Part model, mm, in its own coordinate system. Face numbers are marked on the shaded views. A direction names the side the tool comes from. Give positions to 0.01 mm unless a question says otherwise; leave off trailing zeros. Order: outer loops, then holes, each group sorted by start corner. A loop starts at its lowest first (then second) coordinate and runs counter-clockwise, first axis right, second up. Notation, with made-up numbers: (-32, 55.25) -> (24, 55.25) arc R29 ccw to (24, 91.25) -> close; hole circle Ø11 at (-3.75, 11). An arc over 180 degrees is marked (long way). Write item = value, one per line. Start each with the question number.
Item 1: Band-saw the part on B-B on x = -1.75. Write the cut outline in (y, z), plus the area to 3 significant figures.
Item 2: Band-saw the part on D-D on y = -1.5. Write the cut outline in (x, z).
Item 3: Drill centre lines: line 1 along Z through (x, y) = (4.75, 1.5); line 2 along Z through (x, y) = (8, 3.6); line 3 along X through (y, z) = (3.7, 0). Where is each one in solid material? Low to high.
Item 4: Tool access for the marked faces 4, 5 and 6: list every direction of +Z, -Z, +X, -X, +Y, -Y with a clear straight run to the whole face (end or side of a thin tool).
Item 5: Pull direction Z, two halves, no side cores. Call the marked faces 1, 2 and 3: +Z half, -Z half, draft (parallel to the pull), parting line (faces both ways), or undercut.
Item 6: Band-saw the part on C-C on z = 3. Write the cut outline in (x, y), plus the area to 3 significant figures.
Item 7: Band-saw the part on A-A on y = 0. Write the cut outline in (x, z), plus the area to 3 significant figures.
Item 8: Flat gauge pins, fed straight in: P1, Ø3, axis at y = -3, z = 2, coming from the -X side; P2, Ø2.5, axis at x = 6.5, z = -0.5, coming from the -Y side; P3, Ø3, axis at y = 2.5, z = 2.5, coming from the -X side; P4, Ø0.9, axis at y = 2, z = 1.5, coming from the -X side. Where does each tip first touch, or does it go through?
Autodesk Inventor part; units mm, degrees
ref_plane "Work Plane1" through (0, 0, -2.8) normal (0, 0, -1) x (-1, 0, 0)
ref_plane "Work Plane2" through (8, 0, 0) normal (1, 0, 0) x (0, 1, 0)
ref_plane "XZ Plane" through (0, 0, 0) normal (0, 1, 0) x (-1, 0, 0)
sketch "Sketch1" plane through (0, 0, 0) normal (0, 0, 1) x (1, 0, 0)
  circle A0 centre (0, 0) radius 4
  dimension "d0" = 8
extrude "Extrusion1" add sketch "Sketch1" along normal mid plane 8
sketch "Sketch2" plane through (0, 0, 4) normal (0, 0, 1) x (1, 0, 0)
  circle A0 centre (0, 0) radius 2.4
  line L0 (-2.2627, 0.8) -> (-0.8, 0.8)
  line L1 (-0.8, 0.8) -> (-0.8, 2.2627)
  line L2 (0.8, 2.2627) -> (0.8, 0.8)
  line L3 (0.8, 0.8) -> (2.2627, 0.8)
  line L4 (2.2627, -0.8) -> (0.8, -0.8)
  line L5 (0.8, -0.8) -> (0.8, -2.2627)
  line L6 (-0.8, -2.2627) -> (-0.8, -0.8)
  line L7 (-0.8, -0.8) -> (-2.2627, -0.8)
  dimension "d3" = 4.8
  dimension "d4" = 1.6
extrude "Extrusion2" cut sketch "Sketch2" against normal through all contours A0 L4 L5 L6 L7 L0 L1 L2 L3
ref_plane "Work Plane1" through (0, 0, -2.8) normal (0, 0, -1) x (-1, 0, 0)
sketch "Sketch3" plane through (0, 0, -2.8) normal (0, 0, -1) x (-1, 0, 0)
  circle A0 centre (0, 0) radius 4
  circle A1 centre (0, 0) radius 4
  circle A2 centre (0, 0) radius 3
  dimension "d8" = 6
extrude "Extrusion3" cut sketch "Sketch3" against normal blind 5.6
sketch "Sketch5" plane through (0, 0, 0) normal (0, 1, 0) x (-1, 0, 0)
  line L0 (-0.8, 4) -> (-0.8, -4)
  line L1 (0.8, 4) -> (0.8, -4)
  line L2 (4, 2.8) -> (-4, 2.8)
  line L3 (-0.8, -2.8) -> (0.8, -2.8)
  line L4 (0.8, -2.8) -> (0.8, 2.8)
  line L5 (0.8, 2.8) -> (-0.8, 2.8)
  line L6 (-0.8, 2.8) -> (-0.8, -2.8)
  point P0 (0, 0)
  point P1 (-1.518, -3.6)
  point P2 (4, -2.8)
  point P3 (4, -2.8)
extrude "Extrusion5" cut sketch "Sketch5" along normal through all both and the other way through all
fillet "Fillet1" radius 0.3 16 edges at (-0.8, 0.8, 0) (-0.8, -0.8, 0) (0.8, -0.8, 0) (0.8, 0.8, 0) (-2.2627, -0.8, 0) (-2.2627, 0.8, 0) (-0.8, 2.2627, 3.4) (0.8, 2.2627, 3.4) (2.2627, 0.8, 0) (2.2627, -0.8, 0) (0.8, -2.2627, 3.4) (-0.8, -2.2627, 3.4) (0.8, 2.2627, -3.4) (-0.8, 2.2627, -3.4) (0.8, -2.2627, -3.4) (-0.8, -2.2627, -3.4)
sketch "Sketch6" plane through (0, 0, 0) normal (0, 1, 0) x (-1, 0, 0)
  circle A0 centre (-8, 0) radius 2.5
  circle A1 centre (-8, 0) radius 4
  line L0 (-4, 2.8) -> (-4, 4)
  line L1 (-4, -4) -> (-4, -2.8)
  line L2 (-8, 4) -> (-8, -4) construction
  point P0 (0, 0)
  dimension "d22" = 5
  dimension "d23" = 8
  dimension "d24" = 8
extrude "Extrusion6" add sketch "Sketch6" along normal mid plane 8
sketch "Sketch7" plane through (8, 4, 0) normal (0, 1, 0) x (1, 0, 0)
  circle A0 centre (0, 0) radius 2.5
  circle A1 centre (0, 0) radius 4
  circle A2 centre (0, 0) radius 2.6667
  point P0 (-8, 0)
  dimension "d27" = 5.3333
extrude "Extrusion7" cut sketch "Sketch7" against normal blind 0.5333 contours A2
mirror "Mirror1" about plane through (0, 0, 0) normal (0, 1, 0) of "Extrusion7"
ref_plane "Work Plane2" through (8, 0, 0) normal (1, 0, 0) x (0, 1, 0)
sketch "Sketch8" plane through (8, 0, 0) normal (1, 0, 0) x (0, 1, 0)
  line L0 (-4, -2.6667) -> (-4, 2.6667)
  line L1 (-4, -4) -> (-4, 4)
  line L2 (4, 2.6667) -> (4, -2.6667)
  line L3 (4, 4) -> (4, -4)
  line L4 (4, 4) -> (-4, 4)
  line L5 (-4, 4) -> (-4, 2.8)
  line L6 (-4, 2.8) -> (4, 2.8)
  line L7 (4, 2.8) -> (4, 4)
  line L8 (-4, -4) -> (4, -4)
  line L9 (4, -4) -> (4, -2.8)
  line L10 (4, -2.8) -> (-4, -2.8)
  line L11 (-4, -2.8) -> (-4, -4)
  dimension "d36" = 1.2
extrude "Extrusion8" add sketch "Sketch8" against normal up to surface contours L10 L3 L8 L1 | L1 L4 L3 L6
properties part number "6536" material "Steel"
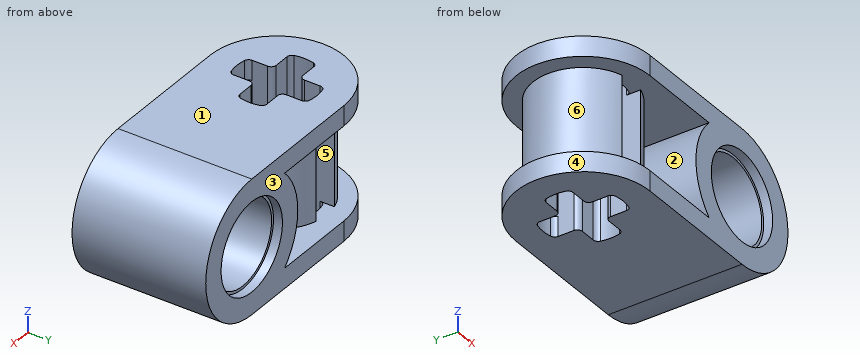
Values found:
q1.outline = (-3.6, -4) -> (-0.8, -4) -> (-0.8, 4) -> (-3.6, 4) -> (-3.6, 2.8) -> (-2.44, 2.8) -> (-2.44, -2.8) -> (-3.6, -2.8) -> close; (0.8, -4) -> (3.6, -4) -> (3.6, -2.8) -> (2.44, -2.8) -> (2.44, 2.8) -> (3.6, 2.8) -> (3.6, 4) -> (0.8, 4) -> close
q1.area = 31.8 mm^2
q2.outline = (-3.71, -4) -> (-0.8, -4) -> (-0.8, 4) -> (-3.71, 4) -> (-3.71, 2.8) -> (-2.6, 2.8) -> (-2.6, -2.8) -> (-3.71, -2.8) -> close; (0.8, -4) -> (8, -4) arc R4 ccw to (8, 4) -> (0.8, 4) -> close; hole (2.6, -2.8) -> (5.14, -2.8) arc R4 cw to (5.14, 2.8) -> (2.6, 2.8) -> close; hole circle Ø5 at (8, 0)
q3.line_1 = -4 to -2.8, -2.33 to 2.33, 2.8 to 4
q3.line_2 = -4 to -2.67, 2.67 to 4
q3.line_3 = 4 to 5.33, 10.67 to 12
q4.face_4 = +Z, -Z, -X
q4.face_5 = none
q4.face_6 = -X
q5.face_1 = +Z half
q5.face_2 = undercut
q5.face_3 = draft
q6.outline = (0, -4) -> (10.65, -4) -> (10.65, 4) -> (0, 4) arc R4 ccw to start; hole (-2.33, -0.57) arc R0.3 ccw to (-2.04, -0.8) -> (-1.1, -0.8) arc R0.3 cw to (-0.8, -1.1) -> (-0.8, -2.04) arc R0.3 ccw to (-0.57, -2.33) arc R2.4 ccw to (0.57, -2.33) arc R0.3 ccw to (0.8, -2.04) -> (0.8, -1.1) arc R0.3 cw to (1.1, -0.8) -> (2.04, -0.8) arc R0.3 ccw to (2.33, -0.57) arc R2.4 ccw to (2.33, 0.57) arc R0.3 ccw to (2.04, 0.8) -> (1.1, 0.8) arc R0.3 cw to (0.8, 1.1) -> (0.8, 2.04) arc R0.3 ccw to (0.57, 2.33) arc R2.4 ccw to (-0.57, 2.33) arc R0.3 ccw to (-0.8, 2.04) -> (-0.8, 1.1) arc R0.3 cw to (-1.1, 0.8) -> (-2.04, 0.8) arc R0.3 ccw to (-2.33, 0.57) arc R2.4 ccw to start
q6.area = 97.8 mm^2
q7.outline = (-4, -4) -> (-2.4, -4) -> (-2.4, 4) -> (-4, 4) -> (-4, 2.8) -> (-3, 2.8) -> (-3, -2.8) -> (-4, -2.8) -> close; (2.4, -4) -> (8, -4) arc R4 ccw to (8, 4) -> (2.4, 4) -> close; hole (3, -2.8) -> (5.14, -2.8) arc R4 cw to (5.14, 2.8) -> (3, 2.8) -> close; hole circle Ø5 at (8, 0)
q7.area = 49.9 mm^2
q8.P1 = -3.61
q8.P2 = -4
q8.P3 = -3.87
q8.P4 = -2.57
